```python
from build123d import *

# Parameters (mm, degrees)
SKETCH1_R                = 300.00000000000006
SKETCH1_R_2              = 75.00000000000001
BOSS_EXTRUDE2_DEPTH      = 300
BOSS_EXTRUDE3_DEPTH      = 0.01
BOSS_EXTRUDE3_DEPTH_BACK = 300
SKETCH2_R                = 75.00000000000003
CUT_EXTRUDE1_DEPTH       = 520.6210158375045
CUT_EXTRUDE1_DEPTH_BACK  = 520.6210158375045
SKETCH3_R                = 30
FILLET1_R                = 10
FILLET2_R                = 10
FILLET3_R                = 10


with BuildPart() as part:
    # Sketch1 → Boss-Extrude2 (new body)
    with BuildSketch(Plane(origin=(0, 0, 0), x_dir=(1, 0, 0), z_dir=(0, 1, 0))):
        with Locations(Location((0, 0, 0), (0, 0, 270))):
            Circle(SKETCH1_R)
        with Locations(Location((0, 0, 0), (0, 0, 270))):
            Circle(SKETCH1_R_2, mode=Mode.SUBTRACT)
    extrude(amount=BOSS_EXTRUDE2_DEPTH)

    # Sketch2 → Boss-Extrude3 (add, two sides: drawn at the far end of the back side and taken through both)
    with BuildSketch(Plane(origin=(0, 300, 0), x_dir=(1, 0, 0), z_dir=(0, 1, 0)).offset(-BOSS_EXTRUDE3_DEPTH_BACK)):
        with Locations(Location((0, 0, 0), (0, 0, 270))):
            Circle(SKETCH2_R)
    extrude(amount=BOSS_EXTRUDE3_DEPTH + BOSS_EXTRUDE3_DEPTH_BACK)

    # Sketch3 → Cut-Extrude1 (cut, two sides: drawn at the far end of the back side and taken through both)
    with BuildSketch(Plane(origin=(0, 300.01, 0), x_dir=(1, 0, 0), z_dir=(0, 1, 0)).offset(-CUT_EXTRUDE1_DEPTH_BACK)):
        with Locations(Location((0, 0, 0), (0, 0, 270))):
            Circle(SKETCH3_R)
    extrude(amount=CUT_EXTRUDE1_DEPTH + CUT_EXTRUDE1_DEPTH_BACK, mode=Mode.SUBTRACT)

    # Fillet1
    # the kernel refuses this fillet: 10 mm, written as the material it takes off along each edge
    with BuildSketch(Plane(origin=(0, 300.01, 0), x_dir=(-1.8e-16, 0, 1), z_dir=(-1, 0, -1.8e-16))) as fillet1_piece_1:
        with BuildLine():
            CenterArc((74.55289822187787, -10), FILLET1_R, 87.43744126687696, 2.5625587331230406)
            Line((74.55289822187787, 0), (75.00000000000003, 0))
            Line((75.00000000000003, 0), (75.00000000000001, -0.00999999999999091))
        make_face()
    revolve(axis=Axis((0, 300.01, 0), (0, 1, 0)), mode=Mode.SUBTRACT)
    with BuildSketch(Plane(origin=(0, 300.01, 0), x_dir=(-1.8e-16, 0, 1), z_dir=(-1, 0, -1.8e-16))) as fillet1_piece_2:
        with BuildLine():
            CenterArc((30 + FILLET1_R, -FILLET1_R), FILLET1_R, 90, 90)
            Line((30 + FILLET1_R, 0), (30, 0))
            Line((30, 0), (30, -FILLET1_R))
        make_face()
    revolve(axis=Axis((0, 300.01, 0), (0, 1, 0)), mode=Mode.SUBTRACT)
    with BuildSketch(Plane(origin=(0, 0, 0), x_dir=(-1.8e-16, 0, 1), z_dir=(-1, 0, -1.8e-16))) as fillet1_piece_3:
        with BuildLine():
            CenterArc((300.00000000000006 - FILLET1_R, FILLET1_R), FILLET1_R, 270, 90)
            Line((300.00000000000006 - FILLET1_R, -1.78e-15), (300.00000000000006, 0))
            Line((300.00000000000006, 0), (300.00000000000006, FILLET1_R))
        make_face()
    revolve(axis=Axis((0, 0, 0), (0, 1, 0)), mode=Mode.SUBTRACT)
    with BuildSketch(Plane(origin=(0, 300, 0), x_dir=(-1.8e-16, 0, 1), z_dir=(-1, 0, -1.8e-16))) as fillet1_piece_4:
        with BuildLine():
            CenterArc((300.00000000000006 - FILLET1_R, -FILLET1_R), FILLET1_R, 0, 90)
            Line((300.00000000000006 - FILLET1_R, 0), (300.00000000000006, 0))
            Line((300.00000000000006, 0), (300.00000000000006, -FILLET1_R))
        make_face()
    revolve(axis=Axis((0, 300, 0), (0, 1, 0)), mode=Mode.SUBTRACT)

    # Fillet2
    # the kernel refuses this fillet: 10 mm, written as the material it adds along each edge
    with BuildSketch(Plane(origin=(0, 300, 0), x_dir=(-1.8e-16, 0, 1), z_dir=(-1, 0, -1.8e-16))) as fillet2_piece_1:
        with BuildLine():
            CenterArc((75.18527469203002, 10), FILLET2_R, 268.1880728619216, 1.8119271380783744)
            ThreePointArc((74.86908645695401, 0.00499999999999545), (74.93455141662679, 0.00271438793976131), (75.00000000000001, 0))
            Line((75.00000000000001, 0), (75.18527469203002, 0))
        make_face()
    revolve(axis=Axis((0, 300, 0), (0, 1, 0)))

    # Fillet3
    fillet3_edges = [part.edges().sort_by_distance(p)[0] for p in [
        (2.251e-14, 0, -30),
    ]]
    fillet(fillet3_edges, radius=FILLET3_R)


solid = part.part
```
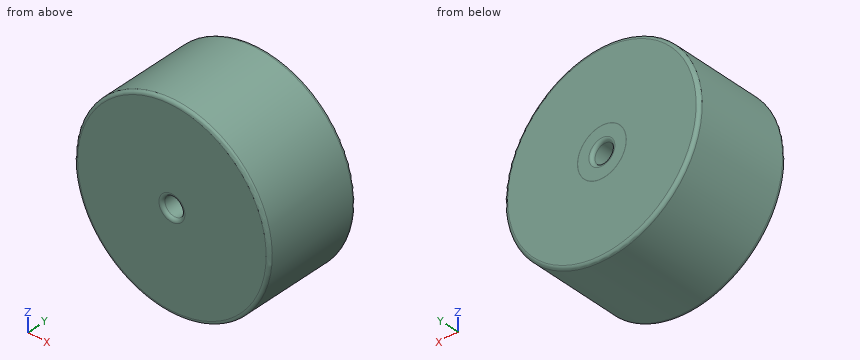
Design review of the part built by this model. Coordinates are the model's own, in mm. Give positions to 0.01 mm unless a question says otherwise; leave off trailing zeros. Order: outer loops, then holes, each group sorted by start corner. A loop starts at its lowest first (then second) coordinate and runs counter-clockwise, first axis right, second up. Notation, with made-up numbers: (35.25, 12.25) - (53.25, 12.25) arc R25 cw to (53.25, 51.25) - close; hole circle Ø6 at (74.25, -12). An arc over 180 degrees is marked (long way). Use a Markdown table: item, result. Add a question column.
(1) Clearance check with flat-ended pins moving along their axes: P1, Ø2, axis at x = 65.5, z = -153, coming from the +Y side; P2, Ø3, axis at y = 182, z = -120, coming from the -X side; P3, Ø6, axis at x = 34.5, y = 91, coming from the -Z side. State where each tip first meets the part, or that it passes through.
(2) Wall thickness on probe 1 along X at (y, z) = (118, 0); probe 2 along Y at (x, z) = (-273.5, 16.5); probe 3 along X at (y, z) = (69, 259.5): over which ranges is each line inside the solid? List them lowest first. Write a range as [from, to].
(3) Add section A-A on y = 124. Give the boundary of the cut face in (x, z).
Report:
| question | item | result |
|---|---|---|
| 1 | P1 | stops at y = 300 |
| 1 | P2 | stops at x = -275.6 |
| 1 | P3 | stops at z = -298.34 |
| 2 | probe 1 | x = [-300, -30], [30, 300] |
| 2 | probe 2 | y = [0, 300] |
| 2 | probe 3 | x = [-150.53, 150.53] |
| 3 | outline | circle Ø600 at (0, 0); hole circle Ø60 at (0, 0) |
